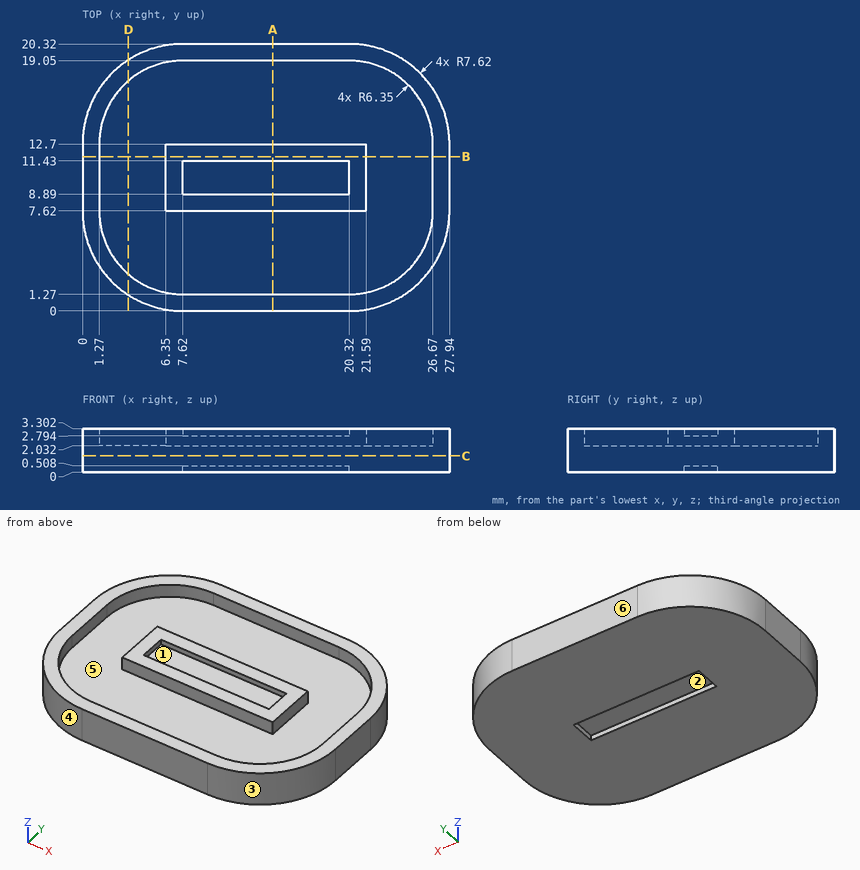
Could you check a few things on this drawing? It's one solid part, dimensions in mm from its lowest x, y, z. A direction names the side the tool comes from. Give positions to 0.01 mm unless a question says otherwise; leave off trailing zeros. Loops run counter-clockwise (first coordinate to the right, second up) from the corner with the lowest first, then second, coordinate; pieces in that order, holes last. Notation, with made-up numbers: M -40,9 L -7,9 A16 cw -7,40 Z; hole C 83,60.25 d2. An arc over 180 degrees is marked long. Answer as a JSON object with one key per item and string values.
Q1. For P1, Ø10, axis at x = 8.5, y = 14.5, coming from the +Z side; P2, Ø1, axis at y = 5.5, z = 1.5, coming from the +X side; P3, Ø0.8, axis at x = 13, y = 10.5, coming from the +Z side, each with a flat end and sliding along its axis, tell me the tip position at first contact or that it passes through.
Values found:
{"P1": "stops at z = 3.3", "P2": "stops at x = 27.77", "P3": "stops at z = 2.79"}
Q2. Suppose I cut it at C-C, the plane z = 1.25. List the corners of the cut face in (x, y) for me.
Values found:
{"outline": "M 0,7.62 A7.62 ccw 7.62,0 L 20.32,0 A7.62 ccw 27.94,7.62 L 27.94,12.7 A7.62 ccw 20.32,20.32 L 7.62,20.32 A7.62 ccw 0,12.7 Z"}
Q3. If I drill on probe 1 along Y at (x, z) = (17.75, 2.45); probe 2 along Y at (x, z) = (10.75, 3.2); probe 3 along X at (y, z) = (10, 2.2), over which ranges is the centre line in solid material (lowest first)? Write a range as [from, to].
Values found:
{"probe 1": "y = [0, 1.27], [7.62, 12.7], [19.05, 20.32]", "probe 2": "y = [0, 1.27], [7.62, 8.89], [11.43, 12.7], [19.05, 20.32]", "probe 3": "x = [0, 1.27], [6.35, 21.59], [26.67, 27.94]"}
Q4. If we mould it in two halves opening along Y, with no side actions, what happens to the marked faces 4, 5 and 6? For each: pulls with the +Y half, pulls with the -Y half, needs draft (parallel to the pull), parting line crosses it, or undercut.
Values found:
{"face 4": "pulls with the -Y half", "face 5": "undercut", "face 6": "pulls with the +Y half"}
Q5. Suppose I cut it at A-A, the plane x = 14.5. List the corners of the cut face in (y, z) for me, plus the area to 3 significant figures.
Values found:
{"outline": "M 0,0 L 8.89,0 L 8.89,0.51 L 11.43,0.51 L 11.43,0 L 20.32,0 L 20.32,3.3 L 19.05,3.3 L 19.05,2.03 L 12.7,2.03 L 12.7,3.3 L 11.43,3.3 L 11.43,2.79 L 8.89,2.79 L 8.89,3.3 L 7.62,3.3 L 7.62,2.03 L 1.27,2.03 L 1.27,3.3 L 0,3.3 Z", "area": "48.4 mm²"}
Q6. Suppose I cut it at D-D, the plane x = 3.5. List the corners of the cut face in (y, z) for me, plus the area to 3 significant figures.
Values found:
{"outline": "M 1.21,0 L 19.11,0 L 19.11,3.3 L 17.53,3.3 L 17.53,2.03 L 2.79,2.03 L 2.79,3.3 L 1.21,3.3 Z", "area": "40.4 mm²"}
Q7. For the marked faces 1, 2 and 3, which set-ups out of +Z, -Z, +X, -X, +Y, -Y let a thin tool reach every point of the face, with its end or its side?
Values found:
{"face 1": "+Z", "face 2": "-Z", "face 3": "+Z, -Z, +X, -Y"}
Q8. Suppose I cut it at B-B, the plane y = 11.75. List the corners of the cut face in (x, z) for me, plus the area to 3 significant figures.
Values found:
{"outline": "M 0,0 L 27.94,0 L 27.94,3.3 L 26.67,3.3 L 26.67,2.03 L 21.59,2.03 L 21.59,3.3 L 6.35,3.3 L 6.35,2.03 L 1.27,2.03 L 1.27,3.3 L 0,3.3 Z", "area": "79.4 mm²"}
